Study the drawing (mm; zero at the part's minimum x, y, z) and answer. Give positions to 0.01 mm unless a question says otherwise; leave off trailing zeros. Loops run counter-clockwise (first coordinate to the right, second up) from the corner with the lowest first, then second, coordinate; pieces in that order, holes last. Notation, with made-up numbers: (42, -39) - (67, -39) arc R24 cw to (67, -6) - close; hole circle Ø4 at (77.25, 75.25). An arc over 180 degrees is marked (long way). Answer in a Markdown table with one row per item. Add a question column.
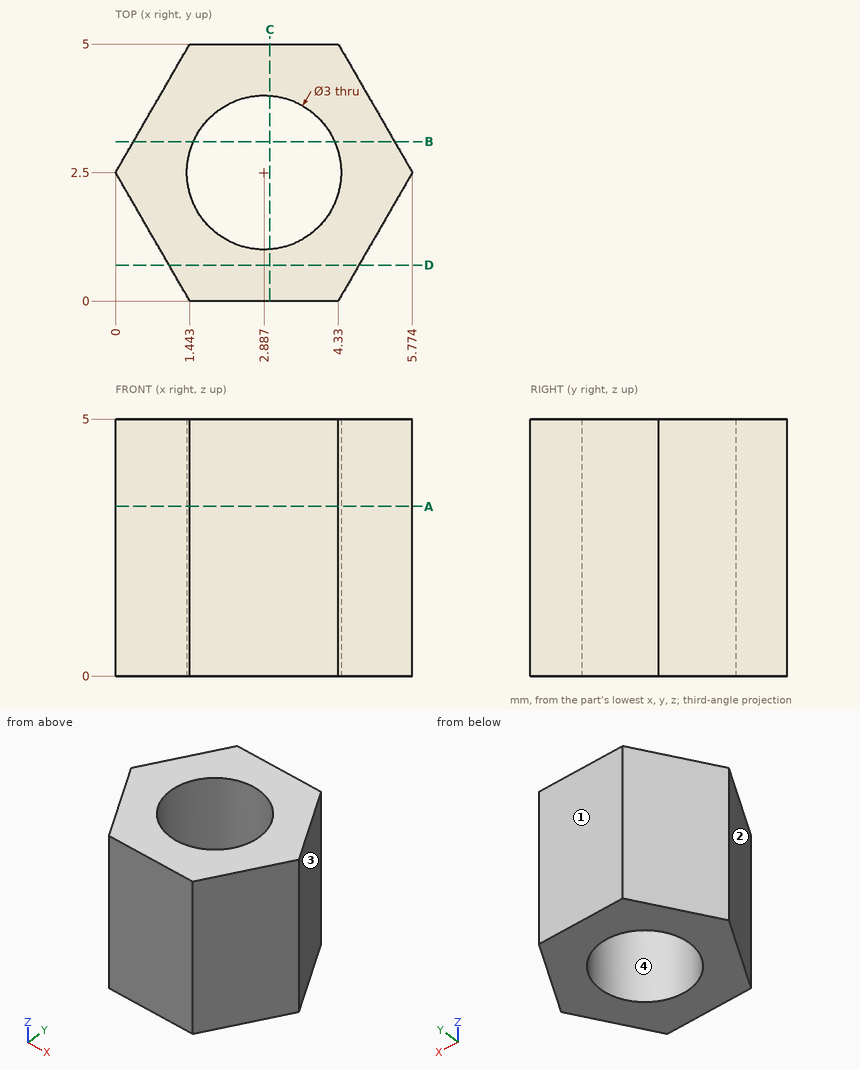
(1) Find the intervals of material crossed by line 1 along Y through (x, z) = (1.65, 2.5); line 2 along Y through (x, z) = (1.8, 0.95) (1 decimal); line 3 along X through (y, z) = (2.4, 1.25) (1 decimal), in increasing order. Write a range as [from, to].
(2) A cutting plane is placed at A-A on z = 3.3. Determine the outline of the cut face in (x, y).
(3) Given pin 1 Ø3 at (y, z) = (1.5, 2) entering from +X, flat-ended and moving along its own axis, determine where the tip first touches the part or whether it passes through.
(4) A cutting plane is placed at D-D on y = 0.7. Determine the outline of the cut face in (x, z) (1 decimal), plus the area to 3 significant figures.
(5) A cutting plane is placed at B-B on y = 3.1. Determine the outline of the cut face in (x, z).
(6) The mould has two halves that part along X. Classify the marked faces 1, 2, 3 and 4: pulls with the +X half, pulls with the -X half, needs draft (parallel to the pull), parting line crosses it, or undercut.
(7) A cutting plane is placed at C-C on x = 3. Determine the outline of the cut face in (y, z) (1 decimal).
Evaluation:
| question | item | result |
|---|---|---|
| 1 | line 1 | y = [0, 1.65], [3.35, 5] |
| 1 | line 2 | y = [0, 1.5], [3.5, 5] |
| 1 | line 3 | x = [0.1, 1.4], [4.4, 5.7] |
| 2 | outline | (0, 2.5) - (1.44, 0) - (4.33, 0) - (5.77, 2.5) - (4.33, 5) - (1.44, 5) - close; hole circle Ø3 at (2.89, 2.5) |
| 3 | pin 1 | stops at x = 5.77 |
| 4 | outline | (1, 0) - (4.7, 0) - (4.7, 5) - (1, 5) - close |
| 4 | area | 18.5 mm² |
| 5 | outline | (0.35, 0) - (1.51, 0) - (1.51, 5) - (0.35, 5) - close; (4.26, 0) - (5.43, 0) - (5.43, 5) - (4.26, 5) - close |
| 6 | face 1 | needs draft |
| 6 | face 2 | pulls with the -X half |
| 6 | face 3 | pulls with the +X half |
| 6 | face 4 | undercut |
| 7 | outline | (0, 0) - (1, 0) - (1, 5) - (0, 5) - close; (4, 0) - (5, 0) - (5, 5) - (4, 5) - close |
